Geometry check sheet. Reference: drawing and pictorial views, mm from the part's lowest x, y, z. A direction names the side the tool comes from. Coordinates: 2 decimals unless noted, no trailing zeros. Loops run counter-clockwise (first coordinate to the right, second up) from the corner with the lowest first, then second, coordinate; pieces in that order, holes last. Notation, with made-up numbers: (37, -27.75) - (44, -27.75) arc R8 cw to (44, -23.75) - close; hole circle Ø9 at (74, -22). An arc over 180 degrees is marked (long way). Use a Markdown table: item, result. Add a question column.
1) Tool access check on the marked faces 1, 2 and 3. Record the directions out of +Z, -Z, +X, -X, +Y, -Y that give a thin tool (end or side, any length) a straight path to the whole face; none if there is none.
2) Sectioned sample at A-A, the plane y = 7.5. Enter the section's corners in (x, z), then the cut area to 3 significant figures.
3) Sectioned sample at B-B, the plane z = 14.5. Enter the section's corners in (x, y).
4) Thickness scan on line 1 (X direction, y = 9.75, z = 29); line 2 (Z direction, x = 40.5, y = 10). Record the ranges inside material, lowest first.
5) Sectioned sample at C-C, the plane x = 9. Enter the section's corners in (y, z), then the cut area to 3 significant figures.
6) Go/stop test with flat-tipped pins: P1, Ø4, axis at y = 9.5, z = 4, coming from the -X side; P2, Ø6, axis at y = 1.5, z = 15, coming from the +X side; P3, Ø4, axis at y = 3, z = 28.5, coming from the -X side. Record where each tip stops, or that it passes through.
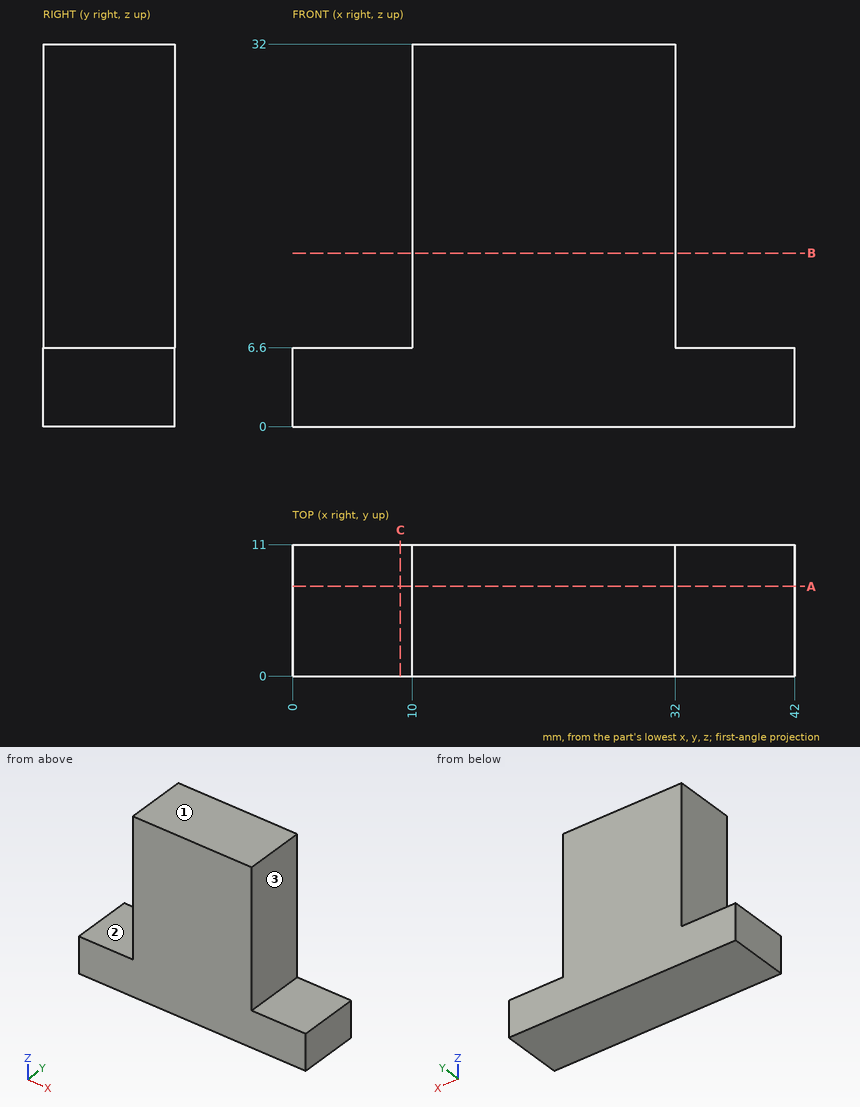
Solved:
| question | item | result |
|---|---|---|
| 1 | face 1 | +Z, +X, -X, +Y, -Y |
| 1 | face 2 | +Z, -X, +Y, -Y |
| 1 | face 3 | +Z, +X, +Y, -Y |
| 2 | outline | (0, 0) - (42, 0) - (42, 6.6) - (32, 6.6) - (32, 32) - (10, 32) - (10, 6.6) - (0, 6.6) - close |
| 2 | area | 836 mm2 |
| 3 | outline | (10, 0) - (32, 0) - (32, 11) - (10, 11) - close |
| 4 | line 1 | x = 10 to 32 |
| 4 | line 2 | z = 0 to 6.6 |
| 5 | outline | (0, 0) - (11, 0) - (11, 6.6) - (0, 6.6) - close |
| 5 | area | 72.6 mm2 |
| 6 | P1 | stops at x = 0 |
| 6 | P2 | stops at x = 32 |
| 6 | P3 | stops at x = 10 |
